from build123d import *

# Parameters (mm, degrees)
CHAMFER1_SIZE = 0.1875
FILLET1_R     = 0.1875


with BuildPart() as part:
    # Sketch3 → Revolve1 (revolve)
    with BuildSketch(Plane(origin=(0, 0, 0), x_dir=(0, 0, -1), z_dir=(1, 0, 0))):
        Polygon((3, 9.5), (0.5, 9.5), (0.5, 7.025), (-3, 7.025), (-3, 4.5), (3, 4.5), align=None)
    revolve(axis=Axis((0, 0, -3), (0, 0, 1)))

    # Chamfer1
    chamfer1_edges = [part.edges().sort_by_distance(p)[0] for p in [
        (0, -4.5, 3),
        (0, -7.025, 3),
        (0, -9.5, -0.5),
        (0, -9.5, -3),
    ]]
    chamfer(chamfer1_edges, length=CHAMFER1_SIZE)

    # Fillet1
    fillet1_edges = [part.edges().sort_by_distance(p)[0] for p in [
        (0, -7.025, -0.5),
    ]]
    fillet(fillet1_edges, radius=FILLET1_R)


solid = part.part
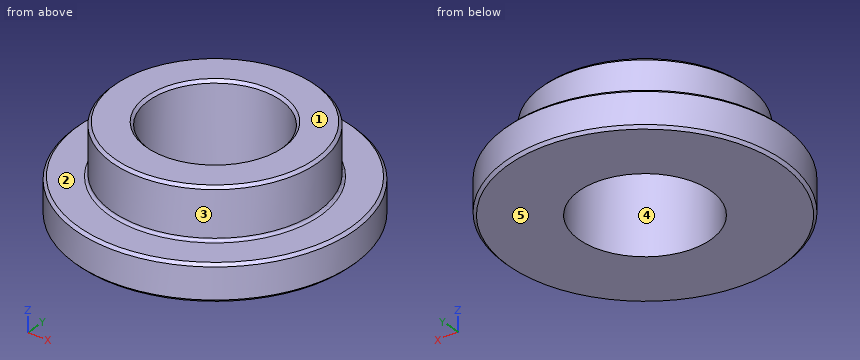
Design review of the part built by this model. Coordinates are the model's own, in mm. Face numbers are marked on the shaded views. A direction names the side the tool comes from. Coordinates: 2 decimals unless noted, no trailing zeros. Order: outer loops, then holes, each group sorted by start corner. A loop starts at its lowest first (then second) coordinate and runs counter-clockwise, first axis right, second up. Notation, with made-up numbers: M 38,51.25 L 53,51.25 A29 ccw 53,82.25 Z; hole C 59,35.5 d1. An arc over 180 degrees is marked long. Use a Markdown table: item, result.
(1) For the marked faces 1 and 2, list the 3-axis set-ups (+Z, -Z, +X, -X, +Y, -Y) from which the entire face can be reached by the end or side of a thin tool; tool diameter is ignored.
Worked answers:
| item | result |
|---|---|
| face 1 | +Z, +X, -X, +Y, -Y |
| face 2 | +Z |
(2) For P1, Ø1, axis at x = 4.5, z = 0.5, coming from the +Y side (3 decimals); P2, Ø1.5, axis at x = 7, z = -2.5, coming from the +Y side; P3, Ø9.5, axis at x = 2, y = -3.5, coming from the +Z side, all flat-tipped, find the tip position at first contact; note any pin that passes through.
Worked answers:
| item | result |
|---|---|
| P1 | stops at y = 5.775 |
| P2 | stops at y = 7.15 |
| P3 | stops at z = 3 |
(3) Add section D-D (z = -2.5). Give the boundary of the cut face in (x, y), then the cut area to 3 significant figures.
Worked answers:
| item | result |
|---|---|
| outline | C 0,0 d19; hole C 0,0 d9 |
| area | 220 mm2 |
(4) Draft analysis for pull direction X (two halves, no side actions). For the marked faces 3, 4 and 5, state which applies: released by +X, released by -X, zero draft, split by the parting line, or undercut.
Worked answers:
| item | result |
|---|---|
| face 3 | split by the parting line |
| face 4 | undercut |
| face 5 | zero draft |
(5) Wall thickness on probe 1 along Y at (x, z) = (0, -0.8); probe 2 along Y at (x, z) = (0, -0.25) (3 decimals): over which ranges is each line inside the solid? List them lowest first.
Worked answers:
| item | result |
|---|---|
| probe 1 | y = -9.5 to -4.5, 4.5 to 9.5 |
| probe 2 | y = -7.025 to -4.5, 4.5 to 7.025 |
(6) Add section C-C (z = 1). Give the boundary of the cut face in (x, y) (3 decimals), then the cut area to 3 significant figures.
Worked answers:
| item | result |
|---|---|
| outline | C 0,0 d14.05; hole C 0,0 d9 |
| area | 91.4 mm2 |
